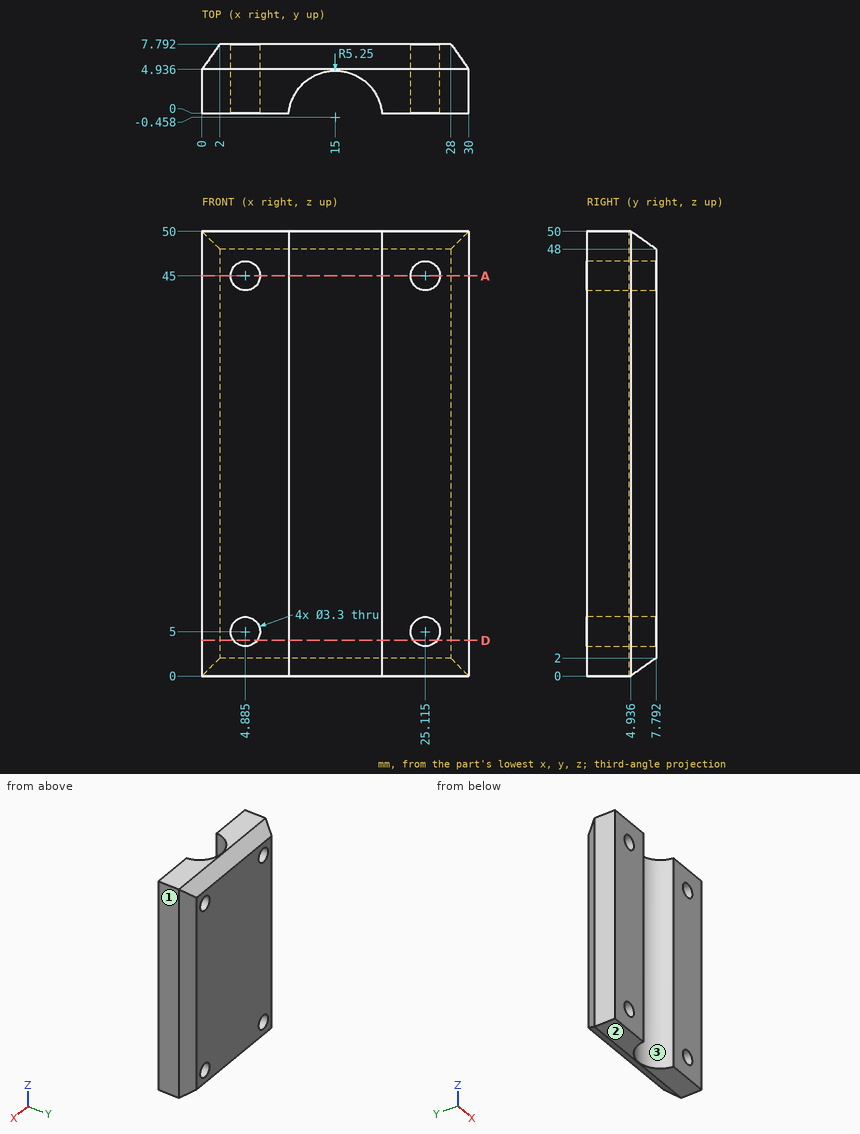
The figure shows three views and two pictorial views of one solid part (mm, origin at its lowest corner). Answer the questions. Round coordinates to 2 decimals unless told otherwise and drop trailing zeros. Loops run counter-clockwise (first coordinate to the right, second up) from the corner with the lowest first, then second, coordinate; pieces in that order, holes last. Notation, with made-up numbers: M 44,51 L 77,51 A32 ccw 77,88 Z; hole C 60.25,48.25 d5. An arc over 180 degrees is marked long. Return JSON: item names as keys, results as strings.
Q1. Find section D-D, the plane z = 4. Determine the outline of the cut face in (x, y), plus the area to 3 significant figures.
Results list:
{"outline": "M 0,0 L 3.57,0 L 3.57,7.79 L 2,7.79 L 0,4.94 Z; M 6.2,0 L 9.77,0 A5.25 cw 20.23,0 L 23.8,0 L 23.8,7.79 L 6.2,7.79 Z; M 26.43,0 L 30,0 L 30,4.94 L 28,7.79 L 26.43,7.79 Z", "area": "149 mm2"}
Q2. Find section A-A, the plane z = 45. State how many separate pieces and enclosed holes the cut face has, plus the area to 3 significant figures.
Results list:
{"separate pieces": "3", "enclosed holes": "0", "area": "138 mm2"}
Q3. The mould has two halves that part along X. Classify the marked faces 1, 2 and 3: released by +X, released by -X, zero draft, split by the parting line, or undercut.
Results list:
{"face 1": "released by +X", "face 2": "zero draft", "face 3": "undercut"}
Q4. Find the intervals of material crossed by line 1 along Z through (x, y) = (24, 0.5) (1 decimal); line 2 along X through (y, z) = (3.75, 45) (1 decimal); line 3 along X through (y, z) = (6.25, 5) (1 decimal), in increasing order. Write a range as from..to.
Results list:
{"line 1": "z = 0..3.8, 6.2..43.8, 46.2..50", "line 2": "x = 0..3.2, 6.5..11.9, 18.1..23.5, 26.8..30", "line 3": "x = 0.9..3.2, 6.5..23.5, 26.8..29.1"}
Q5. Each of these flat-tipped pins is pushed along its axis until it touches: pin 1 Ø1.5 at (x, z) = (12, 8.5) entering from -Y (1 decimal); pin 2 Ø5.5 at (x, z) = (4.88, 45) entering from -Y. Where does it stop, or does it pass through?
Results list:
{"pin 1": "stops at y = 3.2", "pin 2": "stops at y = 0"}
